Check sheet for the modelled part. Datum: model origin and axes. Units: mm. Give positions to 0.01 mm unless a question says otherwise; leave off trailing zeros. Loops run counter-clockwise (first coordinate to the right, second up) from the corner with the lowest first, then second, coordinate; pieces in that order, holes last. Notation, with made-up numbers: (37, 89.5) -> (43, 89.5) arc R12 ccw to (43, 103.5) -> close; hole circle Ø1 at (22, 75). An arc over 180 degrees is marked (long way). Answer as CSV lines item,"result". Start each with the question number.
(1) Material ranges on line 1 (Y direction, x = 1.5, z = 0.05); line 2 (Y direction, x = -0.35, z = 0.95); line 3 (Y direction, x = 1.7, z = 2), recorded low to high. Write a range as from..to.
(2) Section check B-B on x = 0. State how many separate pieces and enclosed holes the cut face has, plus the area to 3 significant figures.
(3) Section check A-A on y = -27. Enter the section's corners in (x, z), plus the area to 3 significant figures.
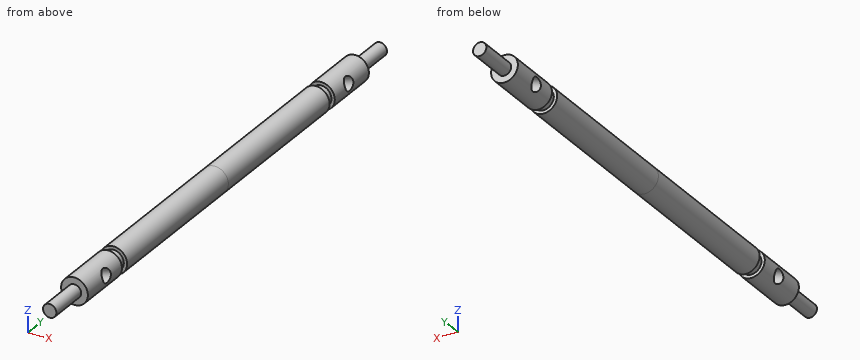
from build123d import *

# Parameters (mm, degrees)
F_2_0MM_PRESS_DOWEL_HOLE1_D = 2.005


with BuildPart() as part:
    # Sketch1 → Revolve1 (revolve)
    with BuildSketch(Plane(origin=(0, 0, 0), x_dir=(0, 0, -1), z_dir=(1, 0, 0))):
        Polygon((-1, 20), (0, 20), (0, 14), (1, 14), (1, 5.75), (0.5, 5.75), (0.5, 4.5), (1, 4.5), (1, -20), (-1, -20), align=None)
    revolve1 = revolve(axis=Axis((0, 20, 1), (0, -1, 0)))

    # Ø2.0mm Press Dowel Hole1 (through all)
    with Locations(Plane(origin=(1.903998662, 9.34, 1.612200209), x_dir=(-0.306100105, 0, 0.951999331), z_dir=(0.951999331, 0, 0.306100105))):
        with Locations((0, 0)):
            f_2_0mm_press_dowel_hole1 = Hole(F_2_0MM_PRESS_DOWEL_HOLE1_D / 2)

    # Mirror1: Revolve1, Ø2.0mm Press Dowel Hole1 across plane
    add(revolve1.mirror(Plane(origin=(0, -20, 1), x_dir=(0, 0, 1), z_dir=(0, 1, 0))))
    add(f_2_0mm_press_dowel_hole1.mirror(Plane(origin=(0, -20, 1), x_dir=(0, 0, 1), z_dir=(0, 1, 0))), mode=Mode.SUBTRACT)


solid = part.part
Working result:
1,line 1,"y = -54..-45.75, -44.5..4.5, 5.75..14"
1,line 2,"y = -60..-50.34, -48.34..8.34, 10.34..20"
1,line 3,"y = -54..-50.24, -48.44..-45.75, -44.5..4.5, 5.75..8.44, 10.24..14"
2,separate pieces,"1"
2,enclosed holes,"2"
2,area,"287 mm^2"
3,outline,"circle Ø4 at (0, 1)"
3,area,"12.6 mm^2"
